```python
from build123d import *

# Parameters (mm, degrees)
F0_W     = 150
F0_H     = 60
F1_DEPTH = 3
F2_W     = 18.75
F2_H     = 3
F3_DEPTH = 3
F4_W     = 3
F4_H     = 15
F5_DEPTH = 3


with BuildPart() as f1:
    # F0 (on Front) → F1 (new body)
    with BuildSketch(Plane.XZ):
        Rectangle(F0_W, F0_H)
    extrude(amount=F1_DEPTH)

    # F2 (on face) → F3 (cut, through all)
    with BuildSketch(Plane.XZ.offset(3)):
        with Locations((-50.125, 28.5)):
            Rectangle(F2_W, F2_H)
        with Locations((-50.125, -1.5)):
            Rectangle(F2_W, F2_H)
        with Locations((0, 28.5)):
            Rectangle(F2_W, F2_H)
        with Locations((0, -1.5)):
            Rectangle(F2_W, F2_H)
        with Locations((50.125, 28.5)):
            Rectangle(F2_W, F2_H)
        with Locations((50.125, -1.5)):
            Rectangle(F2_W, F2_H)
    extrude(amount=-F3_DEPTH, mode=Mode.SUBTRACT)

    # F4 (on face) → F5 (cut, through all)
    with BuildSketch(Plane.XZ.offset(3)):
        with Locations((-73.5, 4.5)):
            Rectangle(F4_W, F4_H)
        with Locations((-73.5, -25.5)):
            Rectangle(F4_W, F4_H)
        with Locations((73.5, 4.5)):
            Rectangle(F4_W, F4_H)
        with Locations((73.5, -25.5)):
            Rectangle(F4_W, F4_H)
    extrude(amount=-F5_DEPTH, mode=Mode.SUBTRACT)


solid = f1.part
```
Model file for the job. Use its own axes, mm. A direction names the side the tool comes from. Give positions to 0.01 mm unless a question says otherwise; leave off trailing zeros. Write each loop counter-clockwise with the first axis right and the second up, starting at its lowest first coordinate (ties: lowest second). Pieces come first, ordered by that corner, then holes. Notation, with made-up numbers: (8, 27.5) -> (39, 27.5) arc R21 cw to (39, 62.5) -> close; hole circle Ø4 at (7.5, -29.75). An arc over 180 degrees is marked (long way). Use CSV: the item, a comma, the result in double quotes. Start each with the question number.
1) Cut at A-A on x = 48.5. List the corners of the cut face in (y, z), plus the area to 3 significant figures.
2) Cut at C-C on y = -2.2. Count the separate pieces of the cut face and the enclosed holes in it, plus the area to 3 significant figures.
3) Pin check, flat tips, straight feed: P1, Ø1.5, axis at x = 3.5, y = -2, coming from the +Z side; P2, Ø1.5, axis at y = -1, z = -1.5, coming from the +X side; P3, Ø3, axis at x = 42.5, z = 13.5, coming from the +Y side. Stop position of each tip, or through.
4) Two-plate mould, pull along X, no slides. Class faces 5 (the flat face through (73, -2, -3)), 6 (the flat face through (75, -1, -11)), 7 (the flat face through (59.5, -2, -2)): released by +X, released by -X, zero draft, split by the parting line, or undercut.
5) Cut at B-B on z = -25. List the corners of the cut face in (x, y).
6) Drill centre lines: L1, parallel to X at y = -0.6, z = 28.5 (3 decimals); L2, parallel to Z at x = -3, y = -1.45; L3, parallel to X at y = -1.85, z = 5. Where is each one in solid material? Low to high.
7) Tool access for faces 1 (the flat face through (59.5, -2, 28)), 2 (the flat face through (72, -2, -24)), 3 (the flat face through (-72, -2, 4)), 4 (the flat face through (0, -2, 0)): list every direction of +Z, -Z, +X, -X, +Y, -Y with a clear straight run to the whole face (end or side of a thin tool).
Final values:
1,outline,"(-3, -30) -> (0, -30) -> (0, -3) -> (-3, -3) -> close; (-3, 0) -> (0, 0) -> (0, 27) -> (-3, 27) -> close"
1,area,"162 mm2"
2,separate pieces,"1"
2,enclosed holes,"3"
2,area,"8,500 mm2"
3,P1,"stops at z = 27"
3,P2,"stops at x = 72"
3,P3,"stops at y = 0"
4,face 5,"zero draft"
4,face 6,"released by +X"
4,face 7,"undercut"
5,outline,"(-72, -3) -> (72, -3) -> (72, 0) -> (-72, 0) -> close"
6,L1,"x = -75 to -59.5, -40.75 to -9.375, 9.375 to 40.75, 59.5 to 75"
6,L2,"z = -30 to -3, 0 to 27"
6,L3,"x = -72 to 72"
7,face 1,"+Z, +Y, -Y"
7,face 2,"-Z, +X, +Y, -Y"
7,face 3,"-X, +Y, -Y"
7,face 4,"+Y, -Y"
